from build123d import *

# Parameters (mm, degrees)
SKETCH1_W           = 90
SKETCH1_H           = 20
SKETCH1_R           = 1.5
BOSS_EXTRUDE1_DEPTH = 3
SKETCH2_W           = 90
SKETCH2_H           = 30
SKETCH2_R           = 1.5
BOSS_EXTRUDE2_DEPTH = 3


with BuildPart() as part:
    # Sketch1 → Boss-Extrude1 (new body)
    with BuildSketch(Plane(origin=(0, 0, 0), x_dir=(1, 0, 0), z_dir=(0, 1, 0))):
        with Locations((31.143497758, 2.511210762)):
            Rectangle(SKETCH1_W, SKETCH1_H)
        with Locations(Location((-6.338089317, 4.011210762, 0), (0, 0, 270))):
            Circle(SKETCH1_R, mode=Mode.SUBTRACT)
        with Locations(Location((66.470970633, 4.011210762, 0), (0, 0, 270))):
            Circle(SKETCH1_R, mode=Mode.SUBTRACT)
    extrude(amount=BOSS_EXTRUDE1_DEPTH)

    # Sketch2 → Boss-Extrude2 (add)
    with BuildSketch(Plane.XY.offset(7.488789238)):
        with Locations((31.143497758, 18)):
            Rectangle(SKETCH2_W, SKETCH2_H)
        with Locations((-10.856502242, 7.5)):
            Circle(SKETCH2_R, mode=Mode.SUBTRACT)
        with Locations((69.743497758, 27.3)):
            Circle(SKETCH2_R, mode=Mode.SUBTRACT)
    extrude(amount=-BOSS_EXTRUDE2_DEPTH)


solid = part.part
Work out the finished part from the listing and answer in its coordinate system (mm). A direction names the side the tool comes from. Round coordinates to 2 decimals unless told otherwise and drop trailing zeros. Loops run counter-clockwise (first coordinate to the right, second up) from the corner with the lowest first, then second, coordinate; pieces in that order, holes last. Notation, with made-up numbers: (82.5, 72.25) - (87.5, 72.25) arc R22 ccw to (87.5, 92.25) - close; hole circle Ø8 at (87, 32). An arc over 180 degrees is marked (long way). One line per item, written item: value.
Q1. Find section D-D on y = 30. Give the vertices of the cut face in (x, z).
Check values:
outline: (-13.86, 4.49) - (76.14, 4.49) - (76.14, 7.49) - (-13.86, 7.49) - close
Q2. Straight lines are drawn through the part: probe 1 along Y at (x, z) = (4, -10); probe 2 along Z at (x, y) = (9.5, 23); probe 3 along X at (y, z) = (8.5, 5.25). For each, find the intervals that lie inside material, in ascending order.
Check values:
probe 1: 0 to 3
probe 2: 4.49 to 7.49
probe 3: -13.86 to -11.97, -9.74 to 76.14
Q3. Find section B-B on x = -2.5. Give the vertices of the cut face in (y, z).
Check values:
outline: (0, -12.51) - (3, -12.51) - (3, 4.49) - (33, 4.49) - (33, 7.49) - (0, 7.49) - close
Q4. For faces 5 (the flat face through (31, 3, -4)), 6 (the flat face through (31, 17, 7.489)), determine the directions among +Z, -Z, +X, -X, +Y, -Y from which every point of the face is accessible in a straight line to the end or side of a thin tool.
Check values:
face 5: -Z, +X, -X, +Y
face 6: +Z, +X, -X, +Y, -Y
Q5. Each of these flat-tipped pins is pushed along its axis until it touches: pin 1 Ø3.5 at (x, z) = (-6.34, -4.01) entering from +Y; pin 2 Ø3.5 at (x, y) = (69.74, 27.3) entering from -Z. Where does it stop, or does it pass through?
Check values:
pin 1: y = 3
pin 2: z = 4.49
Q6. The mould has two halves that part along X. Classify faces 1 (the cylindrical face through (67.736, 1.479, -3.205)), 2 (the flat face through (76.143, 10, 6)), 3 (the cylindrical face through (68.245, 27.366, 6.01)), 4 (the flat face through (31, 18, 4.489)): +X half, -X half, draft (parallel to the pull), parting line (faces both ways), or undercut.
Check values:
face 1: undercut
face 2: +X half
face 3: undercut
face 4: draft
Q7. Find section C-C on z = -7. Give the vertices of the cut face in (x, y).
Check values:
outline: (-13.86, 0) - (76.14, 0) - (76.14, 3) - (-13.86, 3) - close
Q8. Find section A-A on y = 7.5. Give the vertices of the cut face in (x, z), and give its area (3 significant figures).
Check values:
outline: (-13.86, 4.49) - (-12.36, 4.49) - (-12.36, 7.49) - (-13.86, 7.49) - close; (-9.36, 4.49) - (76.14, 4.49) - (76.14, 7.49) - (-9.36, 7.49) - close
area: 261 mm2
